The listing builds one solid part. Answer for the finished solid, in the listing's coordinates (mm). Face numbers are marked on the shaded views. A direction names the side the tool comes from. Round coordinates to 2 decimals unless told otherwise and drop trailing zeros. Write each loop counter-clockwise with the first axis right and the second up, starting at its lowest first coordinate (ties: lowest second). Pieces come first, ordered by that corner, then holes.
Item 1: A tool of negligible diameter and unlimited length cuts with its end or side. For the marked faces 4, 5 and 6, from which of +Z, -Z, +X, -X, +Y, -Y can it reach the whole face along a straight path? Write none if from no direction.
Item 2: Find section D-D on x = -16.5. Give the vertices of the cut face in (y, z), then the cut area to 3 significant figures.
Item 3: For a pull along Y with two mould halves and no side action, classify the marked faces 1, 2 and 3 as +Y half, -Y half, draft (parallel to the pull), parting line (faces both ways), or undercut.
Item 4: Find section C-C on x = -6. Give the vertices of the cut face in (y, z).
Item 5: Find the intervals of material crossed by probe 1 along X at (y, z) = (0, 2); probe 2 along X at (y, z) = (-22.5, 42.5); probe 3 along Y at (x, z) = (3, 12.5), in increasing order.
Item 6: Find section A-A on y = 0. Give the vertices of the cut face in (x, z), then the cut area to 3 significant figures.
Item 7: Each of these flat-tipped pins is pushed along its axis until it touches: pin 1 (12 mm diameter, centred on y = -19.5, z = 20.5, fed in from +X); pin 2 (4 mm diameter, centred on y = -5, z = 49.5, fed in from -X); pin 3 (8 mm diameter, centred on x = -3.5, z = 37, fed in from +Y); pin 4 (6 mm diameter, centred on y = -30.5, z = 43.5, fed in from +X). Where does it stop, or does it pass through?
Item 8: Find section B-B on z = 9. Give the vertices of the cut face in (x, y).
```python
from build123d import *

# Parameters (mm, degrees)
F0_W           = 31
F0_H           = 52
F0_W_2         = 27.5
F0_H_2         = 48
F1_DEPTH       = 60
F0_W_3         = 57
F0_H_3         = 78
F2_DEPTH       = 3
F3_W           = 31
F3_H           = 52
F3_W_2         = 27.5
F3_H_2         = 48
F4_DEPTH       = 3
F5_R           = 5
F6_DEPTH       = 4
F5_R_2         = 6
F7_DEPTH       = 10
F8_R           = 2.5
F9_DEPTH       = 5
F10_R          = 3
F11_W          = 2
F11_H          = 6
F12_DEPTH      = 15
F12_DEPTH_BACK = 15


with BuildPart() as f1:
    # F0 (on Top) → F1 (new body)
    with BuildSketch(Plane.XY):
        with Locations((0.25, 0)):
            Rectangle(F0_W, F0_H)
        Rectangle(F0_W_2, F0_H_2, mode=Mode.SUBTRACT)
    extrude(amount=F1_DEPTH)

    # F0 (on Top) → F2 (join)
    with BuildSketch(Plane.XY):
        Rectangle(F0_W_3, F0_H_3)
        with Locations((0.25, 0)):
            Rectangle(F0_W, F0_H, mode=Mode.SUBTRACT)
    extrude(amount=F2_DEPTH)

    # F3 (on face) → F4 (join)
    with BuildSketch(Plane.XY.offset(60)):
        with Locations((0.25, 0)):
            Rectangle(F3_W, F3_H)
        Rectangle(F3_W_2, F3_H_2, mode=Mode.SUBTRACT)
        Rectangle(F3_W_2, F3_H_2)
    extrude(amount=F4_DEPTH)

    # F5 (on face) → F6 (cut)
    with BuildSketch(Plane.XY.offset(63)):
        with Locations((-4.7345235944, -11.5115633234)):
            Circle(F5_R)
    extrude(amount=-F6_DEPTH, mode=Mode.SUBTRACT)

    # F5 (on face) → F7 (join)
    with BuildSketch(Plane.XY.offset(63)):
        with Locations((-4.7345235944, -11.5115633234)):
            Circle(F5_R_2)
        with Locations((-4.7345235944, -11.5115633234)):
            Circle(F5_R, mode=Mode.SUBTRACT)
    extrude(amount=F7_DEPTH)

    # F8 (on face) → F9 (cut)
    with BuildSketch(Plane.XY):
        with Locations((-20.2327246665, 0)):
            Circle(F8_R)
        with Locations((19.7672753335, 0)):
            Circle(F8_R)
    extrude(amount=F9_DEPTH, mode=Mode.SUBTRACT)

    # F10
    f10_edges = [f1.edges().sort_by_distance(p)[0] for p in [
        (28.5, 39, 1.5),
        (28.5, -39, 1.5),
        (-28.5, 39, 1.5),
        (-28.5, -39, 1.5),
        (-15.25, 26, 33),
        (15.75, 26, 33),
        (-15.25, -26, 33),
        (15.75, -26, 33),
        (15.75, 0, 63),
        (0.25, 26, 63),
        (-15.25, 0, 63),
        (0.25, -26, 63),
    ]]
    fillet(f10_edges, radius=F10_R)

    # F11 (on Right) → F12 (cut, two sides)
    with BuildSketch(Plane.YZ) as f12_sk:
        with Locations((-8.8742363974, 68)):
            Rectangle(F11_W, F11_H)
    extrude(amount=-F12_DEPTH, mode=Mode.SUBTRACT)
    extrude(f12_sk.sketch, amount=F12_DEPTH_BACK, mode=Mode.SUBTRACT)


solid = f1.part
```
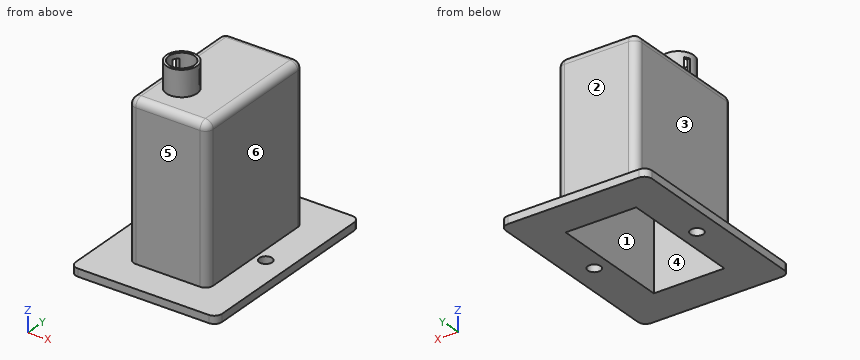
Check values:
1. face 4: -Z
1. face 5: +Z, +X, -X, -Y
1. face 6: +Z, +X, +Y, -Y
2. outline: (-39, 0) - (39, 0) - (39, 3) - (-39, 3) - close
2. area: 234 mm2
3. face 1: undercut
3. face 2: +Y half
3. face 3: draft
4. outline: (-39, 0) - (-24, 0) - (-24, 60) - (-16.35, 60) - (-16.35, 73) - (-17.38, 73) - (-17.38, 63) - (-23, 63) arc R3 ccw to (-26, 60) - (-26, 3) - (-39, 3) - close; (-6.67, 60) - (24, 60) - (24, 0) - (39, 0) - (39, 3) - (26, 3) - (26, 60) arc R3 ccw to (23, 63) - (-5.65, 63) - (-5.65, 73) - (-6.67, 73) - close
5. probe 1: x = -28.5 to -22.73, -17.73 to -13.75, 13.75 to 17.27, 22.27 to 28.5
5. probe 2: x = -15.25 to -13.75, 13.75 to 15.75
5. probe 3: y = -26 to -24, 24 to 26
6. outline: (-28.5, 0) - (-22.73, 0) - (-22.73, 3) - (-28.5, 3) - close; (-17.73, 0) - (-13.75, 0) - (-13.75, 60) - (13.75, 60) - (13.75, 0) - (17.27, 0) - (17.27, 3) - (15.75, 3) - (15.75, 60) arc R3 ccw to (12.75, 63) - (-12.25, 63) arc R3 ccw to (-15.25, 60) - (-15.25, 3) - (-17.73, 3) - close; (22.27, 0) - (28.5, 0) - (28.5, 3) - (22.27, 3) - close
6. area: 347 mm2
7. pin 1: stops at x = 15.75
7. pin 2: stops at x = -15.25
7. pin 3: stops at y = 26
7. pin 4: passes through
8. outline: (-15.25, -23) arc R3 ccw to (-12.25, -26) - (12.75, -26) arc R3 ccw to (15.75, -23) - (15.75, 23) arc R3 ccw to (12.75, 26) - (-12.25, 26) arc R3 ccw to (-15.25, 23) - close; hole (-13.75, -24) - (13.75, -24) - (13.75, 24) - (-13.75, 24) - close
